from build123d import *

# Parameters (mm, degrees)
CROQUIS1_W              = 170
CROQUIS1_H              = 20
CROQUIS1_W_2            = 180
CROQUIS1_H_2            = 16
SALIENTE_EXTRUIR1_DEPTH = 5
CROQUIS2_R              = 1.5
CORTAR_EXTRUIR1_DEPTH   = 106.949338837
CROQUIS3_W              = 170
CROQUIS3_H              = 15
SALIENTE_EXTRUIR2_DEPTH = 5
CROQUIS5_W              = 170
CROQUIS5_H              = 4
CORTAR_EXTRUIR3_DEPTH   = 106.949338837


with BuildPart() as part:
    # Croquis1 → Saliente-Extruir1 (new body)
    with BuildSketch(Plane(origin=(0, 0, 0), x_dir=(1, 0, 0), z_dir=(0, 1, 0))):
        Polygon((90, -28), (85, -28), (-85, -28), (-90, -28), (-90, -55.68), (90, -55.68), align=None)
        with Locations((0, -18)):
            Rectangle(CROQUIS1_W, CROQUIS1_H)
        Rectangle(CROQUIS1_W_2, CROQUIS1_H_2)
    extrude(amount=SALIENTE_EXTRUIR1_DEPTH)

    # Croquis2 → Cortar-Extruir1 (cut, through all)
    with BuildSketch(Plane(origin=(0, 5, 0), x_dir=(1, 0, 0), z_dir=(0, 1, 0))):
        with Locations(Location((-87, 0, 0), (0, 0, 270))):
            Circle(CROQUIS2_R)
        with Locations(Location((-87, -41.84, 0), (0, 0, 270))):
            Circle(CROQUIS2_R)
    cortar_extruir1 = extrude(amount=-CORTAR_EXTRUIR1_DEPTH, mode=Mode.SUBTRACT)

    # Simetría1: Cortar-Extruir1 across plane
    add(cortar_extruir1.mirror(Plane(origin=(0, 0, 0), x_dir=(0, 0, 1), z_dir=(1, 0, 0))), mode=Mode.SUBTRACT)

    # Croquis3 → Saliente-Extruir2 (add)
    with BuildSketch(Plane(origin=(0, 5, 0), x_dir=(1, 0, 0), z_dir=(0, 1, 0))):
        with Locations((0, 15.5)):
            Rectangle(CROQUIS3_W, CROQUIS3_H)
    extrude(amount=-SALIENTE_EXTRUIR2_DEPTH)

    # Croquis5 → Cortar-Extruir3 (cut, through all)
    with BuildSketch(Plane(origin=(0, 5, 0), x_dir=(1, 0, 0), z_dir=(0, 1, 0))):
        with Locations((0, 21)):
            Rectangle(CROQUIS5_W, CROQUIS5_H)
    extrude(amount=-CORTAR_EXTRUIR3_DEPTH, mode=Mode.SUBTRACT)


solid = part.part
Read the model definition and answer for the solid it produces. Units are mm, in the model's axes. A direction names the side the tool comes from. Round coordinates to 2 decimals unless told otherwise and drop trailing zeros. Write each loop counter-clockwise with the first axis right and the second up, starting at its lowest first coordinate (ties: lowest second). Pieces come first, ordered by that corner, then holes. Notation, with made-up numbers: (-37, 56) - (2, 56) arc R35 cw to (2, 94) - close; hole circle Ø4 at (-14.5, 43.5). An arc over 180 degrees is marked (long way). One line per question, with ' | ' between items. Start each with the question number.
1. Find the intervals of material crossed by probe 1 along Z at (x, y) = (87, 1.6); probe 2 along X at (y, z) = (3.7, 41.84); probe 3 along X at (y, z) = (0.7, 41), in increasing order. Write a range as [from, to].
2. For faces 4 (the face through (85, 3, -13)), 5 (the face through (85, 2, 18)), 6 (the face through (-88, 2, 8)), 7 (the face through (-88, 2, -8)), determine the directions among +Z, -Z, +X, -X, +Y, -Y from which every point of the face is accessible in a straight line to the end or side of a thin tool.
3. Section A-A (y = 3.65) is taken. Determine the outline of the cut face in (x, z).
4. Each of these flat-tipped pins is pushed along its axis until it touches: pin 1 (1.5 mm diameter, centred on x = 87.5, y = 3.5, fed in from -Z); pin 2 (1.5 mm diameter, centred on y = 2, z = 19.5, fed in from +X); pin 3 (1.5 mm diameter, centred on y = 3, z = 14, fed in from -X). Where does it stop, or does it pass through?
5. Section B-B (z = -13) is taken. Determine the outline of the cut face in (x, y).
6. For a pull along Z with two mould halves and no side action, classify faces 1 (the face through (-1, 3, -19)), 2 (the face through (-1, 2, 55.68)), 3 (the face through (-85, 2, 18)) as +Z half, -Z half, draft (parallel to the pull), parting line (faces both ways), or undercut.
Filled in:
1) probe 1: [-8, -1.5], [1.5, 8], [28, 40.34], [43.34, 55.68] | probe 2: [-90, -88.5], [-85.5, 85.5], [88.5, 90] | probe 3: [-90, -88.24], [-85.76, 85.76], [88.24, 90]
2) face 4: -Z, +X, +Y, -Y | face 5: +X, +Y, -Y | face 6: -X, +Y, -Y | face 7: -Z, -X, +Y, -Y
3) outline: (-90, -8) - (-85, -8) - (-85, -19) - (85, -19) - (85, -8) - (90, -8) - (90, 8) - (85, 8) - (85, 28) - (90, 28) - (90, 55.68) - (-90, 55.68) - (-90, 28) - (-85, 28) - (-85, 8) - (-90, 8) - close; hole circle Ø3 at (-87, 0); hole circle Ø3 at (-87, 41.84); hole circle Ø3 at (87, 0); hole circle Ø3 at (87, 41.84)
4) pin 1: z = -8 | pin 2: x = 85 | pin 3: x = -85
5) outline: (-85, 0) - (85, 0) - (85, 5) - (-85, 5) - close
6) face 1: -Z half | face 2: +Z half | face 3: undercut
